Can you work these out from the drawing? Everything is in mm from the part's minimum corner. Round coordinates to 2 decimals unless told otherwise and drop trailing zeros. Order: outer loops, then holes, each group sorted by start corner. A loop starts at its lowest first (then second) coordinate and runs counter-clockwise, first axis right, second up. Notation, with made-up numbers: M -39.75,61 L 0.25,61 A27 ccw 0.25,80 Z; hole C 21,79.5 d11. An arc over 180 degrees is marked long. Answer as CSV lines item,"result". Start each with the question number.
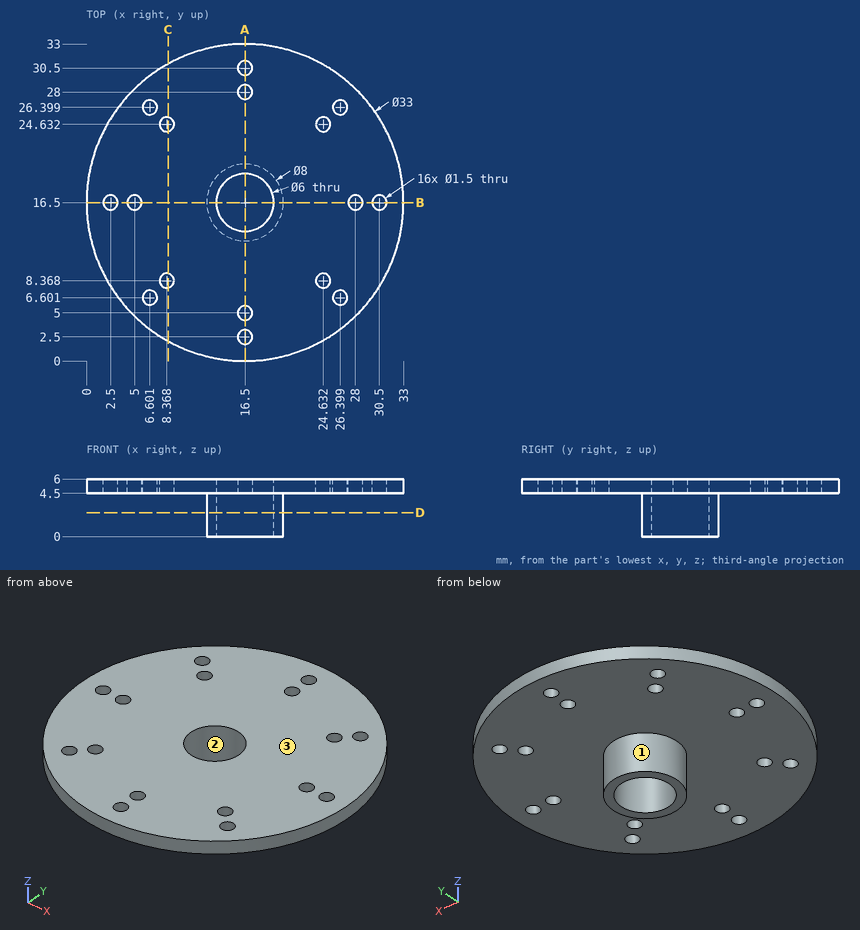
(1) If I drill on line 1 along Y through (x, z) = (16.5, 5.75); line 2 along Y through (x, z) = (19, 2.1) (1 decimal); line 3 along Z through (x, y) = (22, 4.5), over which ranges is the centre line in solid material (lowest first)?
(2) I want a section at D-D on z = 2.5. Write out the boundary of the cut face in (x, y).
(3) I want a section at A-A on x = 16.5. Write out the boundary of the cut face in (y, z).
(4) If we mould it in two halves opening along X, with no side actions, what happens to the marked faces 1, 2 and 3? For each: +X half, -X half, draft (parallel to the pull), parting line (faces both ways), or undercut.
(5) I'm going to push flat-ended pins straight in: P1, Ø1.5, axis at x = 8.5, z = 4, coming from the -Y side; P2, Ø2, axis at x = 26.4, y = 6.6, coming from the -Z side. Where does each tip first touch, or does it pass through?
(6) I want a section at C-C on x = 8.5. Write out the boundary of the cut face in (y, z).
From the geometry:
1,line 1,"0 to 1.75, 3.25 to 4.25, 5.75 to 13.5, 19.5 to 27.25, 28.75 to 29.75, 31.25 to 33"
1,line 2,"13.4 to 14.8, 18.2 to 19.6"
1,line 3,"4.5 to 6"
2,outline,"C 16.5,16.5 d8; hole C 16.5,16.5 d6"
3,outline,"M 0,4.5 L 1.75,4.5 L 1.75,6 L 0,6 Z; M 3.25,4.5 L 4.25,4.5 L 4.25,6 L 3.25,6 Z; M 5.75,4.5 L 12.5,4.5 L 12.5,0 L 13.5,0 L 13.5,6 L 5.75,6 Z; M 19.5,0 L 20.5,0 L 20.5,4.5 L 27.25,4.5 L 27.25,6 L 19.5,6 Z; M 28.75,4.5 L 29.75,4.5 L 29.75,6 L 28.75,6 Z; M 31.25,4.5 L 33,4.5 L 33,6 L 31.25,6 Z"
4,face 1,"parting line"
4,face 2,"undercut"
4,face 3,"draft"
5,P1,"y = 1.77"
5,P2,"z = 4.5"
6,outline,"M 2.07,4.5 L 7.63,4.5 L 7.63,6 L 2.07,6 Z; M 9.11,4.5 L 23.89,4.5 L 23.89,6 L 9.11,6 Z; M 25.37,4.5 L 30.93,4.5 L 30.93,6 L 25.37,6 Z"
